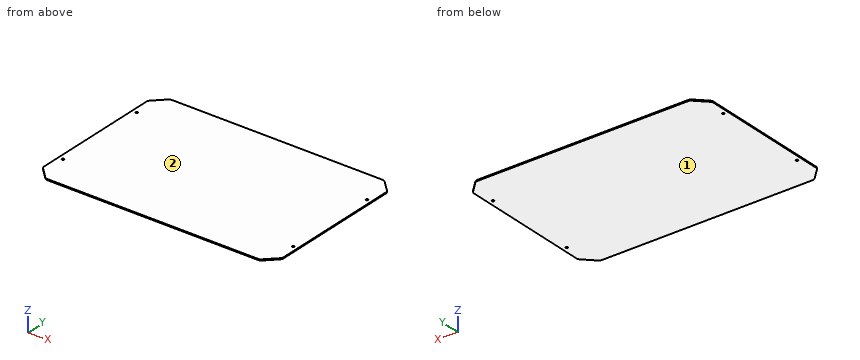
```python
from build123d import *

# Parameters (mm, degrees)
SKETCH2_R           = 4.05
BOSS_EXTRUDE1_DEPTH = 4
FILLET1_R           = 15


with BuildPart() as part:
    # Sketch2 → Boss-Extrude1 (new body)
    with BuildSketch(Plane.XY):
        Polygon((-451.5, 256), (-451.5, -256), (-403.5, -304), (403.5, -304), (451.5, -256), (451.5, 256), (403.5, 304), (-403.5, 304), align=None)
        with Locations((-434, 180)):
            Circle(SKETCH2_R, mode=Mode.SUBTRACT)
        with Locations((-434, -180)):
            Circle(SKETCH2_R, mode=Mode.SUBTRACT)
        with Locations((434, -180)):
            Circle(SKETCH2_R, mode=Mode.SUBTRACT)
        with Locations((434, 180)):
            Circle(SKETCH2_R, mode=Mode.SUBTRACT)
    extrude(amount=BOSS_EXTRUDE1_DEPTH)

    # Fillet1
    fillet1_edges = [part.edges().sort_by_distance(p)[0] for p in [
        (-451.5, -256, 2),
        (-451.5, 256, 2),
        (-403.5, 304, 2),
        (403.5, 304, 2),
        (451.5, 256, 2),
        (451.5, -256, 2),
        (403.5, -304, 2),
        (-403.5, -304, 2),
    ]]
    fillet(fillet1_edges, radius=FILLET1_R)


solid = part.part
```
Can you work these out from the model? Positions are in its coordinate system, mm. Face numbers are marked on the shaded views. Round coordinates to 2 decimals unless told otherwise and drop trailing zeros.
(1) I'm going to push a flat-ended pin straight in: pin 1 (9.5 mm diameter, centred on x = -434, y = -180, fed in from +Z). Where does the tip first touch, or does it pass through?
Results are:
pin 1: stops at z = 4
(2) We'd pull the mould along Z, two halves only. Please class the marked faces 1 and 2: +Z half, -Z half, draft (parallel to the pull), parting line (faces both ways), or undercut.
Results are:
face 1: -Z half
face 2: +Z half
(3) If I drill on L1, parallel to Y at x = -434, z = 1; L2, parallel to X at y = -255.5, z = 3.5, over which ranges is the centre line in solid material (lowest first)?
Results are:
L1: y = -273.5 to -184.05, -175.95 to 175.95, 184.05 to 273.5
L2: x = -450.37 to 450.37
